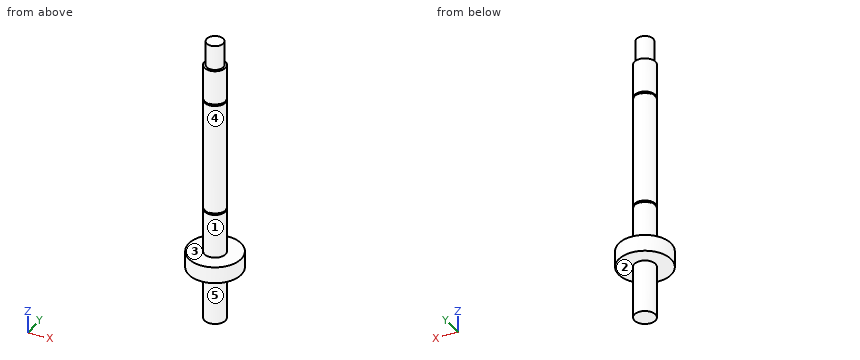
from build123d import *

# Parameters (mm, degrees)
SKETCH1_R           = 6.35
BOSS_EXTRUDE1_DEPTH = 175
CUT_EXTRUDE1_START  = 175
SKETCH2_R           = 8.212767486
SKETCH2_R_2         = 5
CUT_EXTRUDE1_DEPTH  = 15
BOSS_EXTRUDE2_START = 42
SKETCH3_R           = 15.875
BOSS_EXTRUDE2_DEPTH = 10
CUT_EXTRUDE2_START  = 69
SKETCH4_R           = 12.7
SKETCH4_R_2         = 5.715
CUT_EXTRUDE2_DEPTH  = 1.016
CUT_EXTRUDE3_START  = 137.984
SKETCH5_R           = 12.7
SKETCH5_R_2         = 5.715
CUT_EXTRUDE3_DEPTH  = 1.016


with BuildPart() as part:
    # Sketch1 → Boss-Extrude1 (new body)
    with BuildSketch(Plane.XY):
        Circle(SKETCH1_R)
    extrude(amount=BOSS_EXTRUDE1_DEPTH)

    # Sketch2 → Cut-Extrude1 (cut)
    with BuildSketch(Plane.XY.offset(CUT_EXTRUDE1_START)):
        Circle(SKETCH2_R)
        Circle(SKETCH2_R_2, mode=Mode.SUBTRACT)
    extrude(amount=-CUT_EXTRUDE1_DEPTH, mode=Mode.SUBTRACT)

    # Sketch3 → Boss-Extrude2 (add)
    with BuildSketch(Plane.XY.offset(BOSS_EXTRUDE2_START)):
        Circle(SKETCH3_R)
    extrude(amount=-BOSS_EXTRUDE2_DEPTH)

    # Sketch4 → Cut-Extrude2 (cut)
    with BuildSketch(Plane.XY.offset(CUT_EXTRUDE2_START)):
        Circle(SKETCH4_R)
        Circle(SKETCH4_R_2, mode=Mode.SUBTRACT)
    extrude(amount=CUT_EXTRUDE2_DEPTH, mode=Mode.SUBTRACT)

    # Sketch5 → Cut-Extrude3 (cut)
    with BuildSketch(Plane.XY.offset(CUT_EXTRUDE3_START)):
        Circle(SKETCH5_R)
        Circle(SKETCH5_R_2, mode=Mode.SUBTRACT)
    extrude(amount=CUT_EXTRUDE3_DEPTH, mode=Mode.SUBTRACT)


solid = part.part
CAD build for the part. Positions are in the model's coordinates, mm. Face numbers are marked on the shaded views. A direction names the side the tool comes from. Give positions to 0.01 mm unless a question says otherwise; leave off trailing zeros. Loops run counter-clockwise (first coordinate to the right, second up) from the corner with the lowest first, then second, coordinate; pieces in that order, holes last. Notation, with made-up numbers: M -32,24 L 10,24 A29 ccw 10,46 Z; hole C 41,-31.5 d2. An arc over 180 degrees is marked long. One line per question, with ' | ' between items. Start each with the question number.
1. Saw through at C-C on z = 125.5. Give the cut face in (x, y).
2. Flat gauge pins, fed straight in: pin 1 (4 mm diameter, centred on x = 4.5, z = 91, fed in from -Y); pin 2 (1 mm diameter, centred on x = -6.5, y = -10.5, fed in from +Z); pin 3 (4 mm diameter, centred on x = -6.5, z = 39.5, fed in from +Y). Where does each tip first touch, or does it go through?
3. 3-axis set-ups, long thin cutter, end or side, ignore diameter. For the marked faces 4 and 5: which of +Z, -Z, +X, -X, +Y, -Y reach the whole face in a straight line?
4. Saw through at D-D on x = -12.5. Give the cut face in (y, z), plus the area to 3 significant figures.
5. Two-plate mould, pull along Z, no slides. Class the marked faces 1, 2 and 3: pulls with the +Z half, pulls with the -Z half, needs draft (parallel to the pull), parting line crosses it, or undercut.
6. Probe L1, parallel to Z at x = -8, y = -5.5; L2, parallel to X at y = -0.5, z = 91.5; L3, parallel to X at y = -4, z = 22.5. List the from-to ranges inside material, lowest first. Write a range as from..to.
Result sheet:
1) outline: C 0,0 d12.7
2) pin 1: stops at y = -5.84 | pin 2: stops at z = 42 | pin 3: stops at y = 15.22
3) face 4: +Z | face 5: -Z
4) outline: M -9.79,32 L 9.79,32 L 9.79,42 L -9.79,42 Z | area: 196 mm^2
5) face 1: needs draft | face 2: pulls with the -Z half | face 3: pulls with the +Z half
6) L1: z = 32..42 | L2: x = -6.33..6.33 | L3: x = -4.93..4.93
